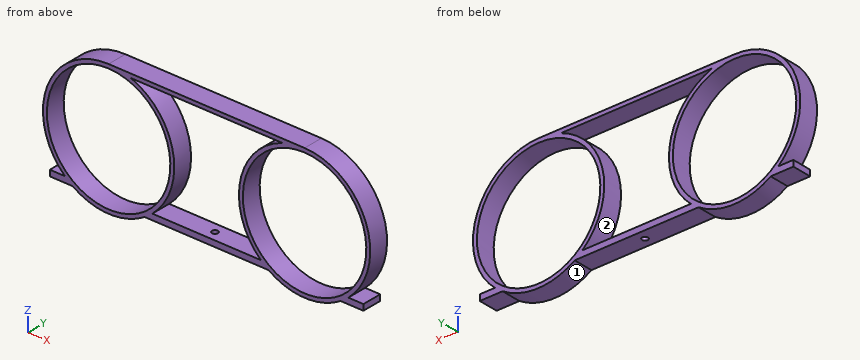
```python
from build123d import *

# Parameters (mm, degrees)
SKETCH3_R           = 31.5
BOSS_EXTRUDE5_DEPTH = 10
SKETCH4_R           = 1.5
CUT_EXTRUDE1_DEPTH  = 22


with BuildPart() as part:
    # Sketch3 → Boss-Extrude5 (new body)
    with BuildSketch(Plane(origin=(0, 0, 0), x_dir=(1, 0, 0), z_dir=(0, 1, 0))):
        with BuildLine():
            Line((-30, 28), (-18.391574158, 28))
            ThreePointArc((-18.391574158, 28), (0, 33.5), (18.391574158, 28))
            Line((18.391574158, 28), (81.608425842, 28))
            ThreePointArc((81.608425842, 28), (100, 33.5), (118.391574158, 28))
            Line((118.391574158, 28), (130, 28))
            Line((130, 28), (130, 25))
            Line((130, 25), (122.299103121, 25))
            ThreePointArc((122.299103121, 25), (131.302955132, -11.932099564), (100, -33.5))
            Line((100, -33.5), (0, -33.5))
            ThreePointArc((0, -33.5), (-31.302955132, -11.932099564), (-22.299103121, 25))
            Line((-22.299103121, 25), (-30, 25))
            Line((-30, 25), (-30, 28))
        make_face()
        with Locations(Location((0, 0, 0), (0, 0, 270))):
            Circle(SKETCH3_R, mode=Mode.SUBTRACT)
        with Locations(Location((100, 0, 0), (0, 0, 270))):
            Circle(SKETCH3_R, mode=Mode.SUBTRACT)
        with BuildLine():
            Line((22.299103121, 25), (77.700896879, 25))
            ThreePointArc((77.700896879, 25), (67.106240001, -6.34433236), (88.598245749, -31.5))
            Line((88.598245749, -31.5), (11.401754251, -31.5))
            ThreePointArc((11.401754251, -31.5), (32.893759999, -6.34433236), (22.299103121, 25))
        make_face(mode=Mode.SUBTRACT)
    extrude(amount=BOSS_EXTRUDE5_DEPTH)

    # Sketch4 → Cut-Extrude1 (cut)
    with BuildSketch(Plane(origin=(0, 0, -28), x_dir=(-1, 0, 0), z_dir=(0, 0, -1))):
        with Locations((-50, 5)):
            Circle(SKETCH4_R)
    extrude(amount=-CUT_EXTRUDE1_DEPTH, mode=Mode.SUBTRACT)


solid = part.part
```
Build history of the part. All positions in model axes, mm. Face numbers are marked on the shaded views. Round coordinates to 2 decimals unless told otherwise and drop trailing zeros. Loops run counter-clockwise (first coordinate to the right, second up) from the corner with the lowest first, then second, coordinate; pieces in that order, holes last.
Item 1: Saw through at D-D (z = 18.5). List the corners of the cut face in (x, y), then the cut area to 3 significant figures.
Item 2: Drill centre lines: line 1 along X through (y, z) = (7, 0); line 2 along X through (y, z) = (3.25, -20.5); line 3 along Y through (x, z) = (50, -26.45). Where is each one in solid material? Low to high.
Item 3: Saw through at B-B (y = 8). List the corners of the cut face in (x, z), then the cut area to 3 significant figures.
Item 4: Saw through at A-A (x = 50). List the corners of the cut face in (y, z).
Item 5: Two-plate mould, pull along Z, no slides. Class the marked faces 1 and 2: released by +Z, released by -Z, zero draft, split by the parting line, or undercut.
Item 6: Saw through at C-C (z = 0). List the corners of the cut face in (x, y).
Item 7: Pin check, flat tips, straight feed: P1, Ø4, axis at y = 4, z = -26, coming from the -X side; P2, Ø3, axis at y = 1.5, z = -14.5, coming from the +X side; P3, Ø2.5, axis at x = 127.5, y = 3, coming from the +Z side. Stop position of each tip, or through.
Worked answers:
1. outline: (-27.93, 0) - (-25.5, 0) - (-25.5, 10) - (-27.93, 10) - close; (25.5, 0) - (27.93, 0) - (27.93, 10) - (25.5, 10) - close; (72.07, 0) - (74.5, 0) - (74.5, 10) - (72.07, 10) - close; (125.5, 0) - (127.93, 0) - (127.93, 10) - (125.5, 10) - close
1. area: 97.3 mm2
2. line 1: x = -33.5 to -31.5, 31.5 to 33.5, 66.5 to 68.5, 131.5 to 133.5
2. line 2: x = -26.5 to -23.92, 23.92 to 26.5, 73.5 to 76.08, 123.92 to 126.5
2. line 3: y = 0 to 3.5, 6.5 to 10
3. outline: (-30, -28) - (-18.39, -28) arc R33.5 ccw to (18.39, -28) - (81.61, -28) arc R33.5 ccw to (118.39, -28) - (130, -28) - (130, -25) - (122.3, -25) arc R33.5 ccw to (100, 33.5) - (0, 33.5) arc R33.5 ccw to (-22.3, -25) - (-30, -25) - close; hole circle Ø63 at (0, 0); hole (11.4, 31.5) arc R33.5 cw to (22.3, -25) - (77.7, -25) arc R33.5 cw to (88.6, 31.5) - close; hole circle Ø63 at (100, 0)
3. area: 1,220 mm2
4. outline: (0, -28) - (3.5, -28) - (3.5, -25) - (0, -25) - close; (0, 31.5) - (10, 31.5) - (10, 33.5) - (0, 33.5) - close; (6.5, -28) - (10, -28) - (10, -25) - (6.5, -25) - close
5. face 1: released by -Z
5. face 2: undercut
6. outline: (-33.5, 0) - (-31.5, 0) - (-31.5, 10) - (-33.5, 10) - close; (31.5, 0) - (33.5, 0) - (33.5, 10) - (31.5, 10) - close; (66.5, 0) - (68.5, 0) - (68.5, 10) - (66.5, 10) - close; (131.5, 0) - (133.5, 0) - (133.5, 10) - (131.5, 10) - close
7. P1: stops at x = -30
7. P2: stops at x = 130.87
7. P3: stops at z = 20.81
